```python
from build123d import *

# Parameters (mm, degrees)
F1_R          = 2.7
F2_R          = 2.95
F7_DEPTH      = 4.2010331125
F7_DEPTH_BACK = 4.2010331125
F8_R          = 0.4


with BuildPart() as f3:
    # F1 (on Top) → F3 section 0
    with BuildSketch(Plane.XY):
        Circle(F1_R)
    # F2 (on offset) → F3 section 1
    with BuildSketch(Plane.XY.offset(10)):
        Circle(F2_R)
    loft()

    # F4 (on Right) → F5 (revolve)
    with BuildSketch(Plane.YZ):
        with BuildLine():
            Line((-4.2, 10), (0, 10))
            Line((0, 10), (0, 20))
            Line((0, 20), (-2.5, 20))
            ThreePointArc((-2.5, 20), (-3.7757084126, 15.0723704301), (-4.2, 10))
        make_face()
    revolve(axis=Axis((0, 0, 5), (0, 0, -1)))

    # F6 (on Right) → F7 (cut, two sides)
    with BuildSketch(Plane.YZ) as f7_sk:
        with BuildLine():
            Line((0.9, 20), (-0.9, 20))
            Line((-0.9, 20), (-0.9, 19.6))
            Line((-0.9, 19.6), (-1.0490520763, 16.0946065159))
            ThreePointArc((-1.0490520763, 16.0946065159), (0, 15), (1.0490520763, 16.0946065159))
            Line((1.0490520763, 16.0946065159), (0.9, 19.6))
            Line((0.9, 19.6), (0.9, 20))
        make_face()
    extrude(amount=-F7_DEPTH, mode=Mode.SUBTRACT)
    extrude(f7_sk.sketch, amount=F7_DEPTH_BACK, mode=Mode.SUBTRACT)

    # F8
    f8_edges = [f3.edges().sort_by_distance(p)[0] for p in [
        (1.414214, -2.061553, 20),
        (-1.414214, -2.061553, 20),
        (0, 2.5, 20),
    ]]
    fillet(f8_edges, radius=F8_R)


solid = f3.part
```
The listing builds one solid part. Answer for the finished solid, in the listing's coordinates (mm). A direction names the side the tool comes from. Coordinates: 2 decimals unless noted, no trailing zeros. Loops run counter-clockwise (first coordinate to the right, second up) from the corner with the lowest first, then second, coordinate; pieces in that order, holes last. Notation, with made-up numbers: M 34.5,-1.75 L 64.5,-1.75 A21 cw 64.5,3.25 Z; hole C -11,53.5 d2. An arc over 180 degrees is marked long. Answer as CSV lines item,"result". Start each with the question number.
(1) Find the intervals of material crossed by L1, parallel to X at y = 1.75, z = 18; L2, parallel to Y at x = -0.5, z = 17.25; L3, parallel to X at y = -1.75, z = 6.75, in increasing order. Write a range as [from, to].
(2) The part is cut by section A-A (z = 7.5). Give the vertices of the cut face in (x, y) (1 decimal), and give its area (3 significant figures).
(3) The part is cut by section B-B (z = 5). Give the vertices of the cut face in (x, y) (3 decimals), and give its area (3 significant figures).
(4) Given pin 1 (1 mm diameter, centred on y = 2, z = 10, fed in from +X); pin 2 (4 mm diameter, centred on x = 2.5, z = 8.5, fed in from -Y); pin 3 (1.5 mm diameter, centred on y = -2.5, z = 15, fed in from +X), each flat-ended and moving along its own axis, determine where each tip first touches the part or whether it passes through.
(5) The mould has two halves that part along Y. Classify faces 4 (the flat face through (0, 1.5, 20)), 5 (the flat face through (-0.048, -0.973, 17.872)), 6 (the conical face through (-0.4, 2.8, 5.1)), 7 (the cylindrical face through (0, 0, 15)): pulls with the +Y half, pulls with the -Y half, needs draft (parallel to the pull), parting line crosses it, or undercut.
(6) For faces 1 (the flat face through (1, 3, 10)), 2 (the flat face through (-0.048, 0.976, 17.823)), 3 (the flat face through (0, 0, 0)), determine the directions among +Z, -Z, +X, -X, +Y, -Y from which every point of the face is accessible in a straight line to the end or side of a thin tool.
Determined:
1,L1,"[-2.59, 2.59]"
1,L2,"[-3.28, -1], [1, 3.28]"
1,L3,"[-2.27, 2.27]"
2,outline,"C 0,0 d5.8"
2,area,"26.2 mm2"
3,outline,"C 0,0 d5.65"
3,area,"25.1 mm2"
4,pin 1,"x = 3.92"
4,pin 2,"y = -4.03"
4,pin 3,"x = 3.38"
5,face 4,"needs draft"
5,face 5,"undercut"
5,face 6,"parting line crosses it"
5,face 7,"undercut"
6,face 1,"-Z"
6,face 2,"+X, -X"
6,face 3,"-Z, +X, -X, +Y, -Y"
